```python
from build123d import *

# Parameters (mm, degrees)
SKETCH1_W           = 192.5
SKETCH1_H           = 150
BOSS_EXTRUDE1_DEPTH = 7.5
SKETCH2_W           = 7.5
SKETCH2_H           = 150
BOSS_EXTRUDE2_DEPTH = 92.5
SKETCH3_R           = 2.5
CUT_EXTRUDE1_DEPTH  = 92.5


with BuildPart() as part:
    # Sketch1 → Boss-Extrude1 (new body)
    with BuildSketch(Plane(origin=(0, 0, 0), x_dir=(1, 0, 0), z_dir=(0, 1, 0))):
        with Locations((103.75, 75)):
            Rectangle(SKETCH1_W, SKETCH1_H)
    extrude(amount=BOSS_EXTRUDE1_DEPTH)

    # Sketch2 → Boss-Extrude2 (add)
    with BuildSketch(Plane(origin=(0, 7.5, 0), x_dir=(1, 0, 0), z_dir=(0, 1, 0))):
        with Locations((11.25, 75)):
            Rectangle(SKETCH2_W, SKETCH2_H)
    extrude(amount=BOSS_EXTRUDE2_DEPTH)

    # Sketch3 → Cut-Extrude1 (cut)
    with BuildSketch(Plane.XZ):
        with Locations((188.75, -3.75)):
            Circle(SKETCH3_R)
        with Locations((196.25, -11.25)):
            Circle(SKETCH3_R)
    extrude(amount=-CUT_EXTRUDE1_DEPTH, mode=Mode.SUBTRACT)


solid = part.part
```
The listing builds one solid part. Answer for the finished solid, in the listing's coordinates (mm). A direction names the side the tool comes from. Coordinates: 2 decimals unless noted, no trailing zeros. Order: outer loops, then holes, each group sorted by start corner. A loop starts at its lowest first (then second) coordinate and runs counter-clockwise, first axis right, second up. Notation, with made-up numbers: M -5.75,-18 L 44.25,-18 A28 cw 44.25,11 Z; hole C 57,71.5 d5. An arc over 180 degrees is marked long. Answer as a JSON object with one key per item and string values. Group by question number.
1. Section C-C on z = -92 is taken. Write down the section's boundary in (x, y).
2. Section D-D on y = 70 is taken. Write down the section's boundary in (x, z), then the cut area to 4 significant figures.
3. Section B-B on z = -3.75 is taken. Write down the section's boundary in (x, y), then the cut area to 3 significant figures.
4. Section A-A on x = 188.75 is taken. Write down the section's boundary in (y, z), then the cut area to 3 significant figures.
5. Straight lines are drawn through the part: line 1 (Y direction, x = 91, z = -36); line 2 (X direction, y = 13, z = -59); line 3 (Z direction, x = 188, y = 3). For each, find the intervals that lie inside material, in ascending order.
6. Flat-ended cylindrical pins translate along their axes: P1, Ø10, axis at x = 135.5, z = -66, coming from the -Y side; P2, Ø4, axis at x = 196.25, z = -11.25, coming from the -Y side; P3, Ø5, axis at x = 166, z = -83, coming from the +Y side; P4, Ø10, axis at y = 44, z = -65, coming from the +X side. Find the tip coordinate at first contact, or state that the pin passes through.
7. Determine the mould class of faces 1 (the flat face through (75, 5, -150)), 2 (the flat face through (15, 53, -74)), 3 (the cylindrical face through (191.135, 3.698, -2.999)) for opening direction Z: released by +Z, released by -Z, zero draft, split by the parting line, or undercut.
8. A tool of negligible diameter and unlimited length cuts with its end or side. For faces 4 (the flat face through (106, 7.5, -76)), 5 (the flat face through (102, 0, -76)), from which of +Z, -Z, +X, -X, +Y, -Y can it reach the whole face along a straight path? Write none if from no direction.
Values follow:
{
 "1": {"outline": "M 7.5,0 L 200,0 L 200,7.5 L 15,7.5 L 15,100 L 7.5,100 Z"},
 "2": {"outline": "M 7.5,-150 L 15,-150 L 15,0 L 7.5,0 Z", "area": "1,125 mm2"},
 "3": {"outline": "M 7.5,0 L 186.25,0 L 186.25,7.5 L 15,7.5 L 15,100 L 7.5,100 Z; M 191.25,0 L 200,0 L 200,7.5 L 191.25,7.5 Z", "area": "2,100 mm2"},
 "4": {"outline": "M 0,-150 L 7.5,-150 L 7.5,-6.25 L 0,-6.25 Z; M 0,-1.25 L 7.5,-1.25 L 7.5,0 L 0,0 Z", "area": "1,090 mm2"},
 "5": {"line 1": "0 to 7.5", "line 2": "7.5 to 15", "line 3": "-150 to -6.13, -1.37 to 0"},
 "6": {"P1": "y = 0", "P2": "through", "P3": "y = 7.5", "P4": "x = 15"},
 "7": {"face 1": "released by -Z", "face 2": "zero draft", "face 3": "undercut"},
 "8": {"face 4": "+Z, -Z, +X, +Y", "face 5": "+Z, -Z, +X, -X, -Y"}
}
